from build123d import *

# Parameters (mm, degrees)
SALIENTE_EXTRUIR1_DEPTH = 6
REDONDEO1_R             = 10
REDONDEO2_R             = 5
REDONDEO3_R             = 1
CROQUIS2_R              = 1.803309478
CORTAR_EXTRUIR1_DEPTH   = 6
MATRIZL1_COUNT          = 2
MATRIZL1_PITCH          = 10
MATRIZL2_COUNT          = 2
MATRIZL2_PITCH          = 10


with BuildPart() as part:
    # Croquis1 → Saliente-Extruir1 (new body)
    with BuildSketch(Plane(origin=(0, 0, 0), x_dir=(1, 0, 0), z_dir=(0, 1, 0))):
        Polygon((0, -36.6), (0, -28.6), (7.646653433, -28.6), (7.646653433, -30.6), (22, -30.6), (22, -28.6), (22, 1.6), (22, 3.6), (9.500929434, 3.6), (9.500929434, 1.6), (0, 1.6), (0, 11.6), (30, 11.6), (30, -36.6), align=None)
    extrude(amount=SALIENTE_EXTRUIR1_DEPTH)

    # Redondeo1
    redondeo1_edges = [part.edges().sort_by_distance(p)[0] for p in [
        (30, 3, -11.6),
        (30, 3, 36.6),
    ]]
    fillet(redondeo1_edges, radius=REDONDEO1_R)

    # Redondeo2
    redondeo2_edges = [part.edges().sort_by_distance(p)[0] for p in [
        (22, 3, 30.6),
        (22, 3, -3.6),
    ]]
    fillet(redondeo2_edges, radius=REDONDEO2_R)

    # Redondeo3
    redondeo3_edges = [part.edges().sort_by_distance(p)[0] for p in [
        (0, 3, 28.6),
        (0, 3, -1.6),
    ]]
    fillet(redondeo3_edges, radius=REDONDEO3_R)

    # Croquis2 → Cortar-Extruir1 (cut)
    with BuildSketch(Plane(origin=(0, 6, 0), x_dir=(1, 0, 0), z_dir=(0, 1, 0))):
        with Locations(Location((26, -13.5, 0), (0, 0, 270))):
            Circle(CROQUIS2_R)
    cortar_extruir1 = extrude(amount=-CORTAR_EXTRUIR1_DEPTH, mode=Mode.SUBTRACT)

    # MatrizL1: Cortar-Extruir1 ×2
    with Locations(*[(0, 0, i * MATRIZL1_PITCH) for i in range(1, MATRIZL1_COUNT)]):
        add(cortar_extruir1, mode=Mode.SUBTRACT)

    # MatrizL2: Cortar-Extruir1 ×2
    with Locations(*[(0, 0, -i * MATRIZL2_PITCH) for i in range(1, MATRIZL2_COUNT)]):
        add(cortar_extruir1, mode=Mode.SUBTRACT)


solid = part.part
Build history of the part. All positions in model axes, mm. A direction names the side the tool comes from. Coordinates: 2 decimals unless noted, no trailing zeros. Order: outer loops, then holes, each group sorted by start corner. A loop starts at its lowest first (then second) coordinate and runs counter-clockwise, first axis right, second up. Notation, with made-up numbers: (2.5, 78.25) - (6.5, 78.25) arc R13 cw to (6.5, 83.25) - close; hole circle Ø3 at (49, 85). An arc over 180 degrees is marked (long way). Write item = value, one per line. Start each with the question number.
1) Wall check: line 1 along Z through (x, y) = (15.75, 4.3); line 2 along Z through (x, y) = (25, 5.2); line 3 along X through (y, z) = (2.05, 3.5). Give the ranges that are in metal, low to high. Write a range as from..to.
2) Saw through at B-B on y = 2.35. Write the cut outline in (x, z), then the cut area to 3 significant figures.
3) Saw through at C-C on x = 6. Write the cut outline in (y, z).
4) Saw through at A-A on x = 26. Write the cut outline in (y, z), then the cut area to 3 significant figures.
5) 3-axis set-ups, long thin cutter, end or side, ignore diameter. For faces 1 (the face through (0.301, 3.042, 28.885)), 2 (the face through (26.99, 3.04, -8.75)), 3 (the face through (13, 3, -3.6)): which of +Z, -Z, +X, -X, +Y, -Y reach the whole face in a straight line?
6) Saw through at D-D on z = 23.5. Write the cut outline in (x, y).
7) Flat gauge pins, fed straight in: pin 1 Ø3 at (x, y) = (25.5, 4) entering from +Z; pin 2 Ø6 at (x, z) = (12.5, 25) entering from -Y; pin 3 Ø3 at (y, z) = (2.5, 12.5) entering from -X; pin 4 Ø1.5 at (y, z) = (4, -1.5) entering from -X. Where does each tip first touch, or does it go through?
8) Two-plate mould, pull along X, no slides. Class faces 4 (the face through (22, 3, 13)), 5 (the face through (9.501, 3, -3)), 6 (the face through (25, 0, 7)): pulls with the +X half, pulls with the -X half, needs draft (parallel to the pull), parting line crosses it, or undercut.
From the geometry:
q1.line_1 = -11.6..-3.6, 30.6..36.6
q1.line_2 = -10.26..2, 5..12, 15..22, 25..35.26
q1.line_3 = 22..24.2, 27.8..30
q2.outline = (0, -11.6) - (20, -11.6) arc R10 ccw to (30, -1.6) - (30, 26.6) arc R10 ccw to (20, 36.6) - (0, 36.6) - (0, 29.6) arc R1 ccw to (1, 28.6) - (7.65, 28.6) - (7.65, 30.6) - (17, 30.6) arc R5 cw to (22, 25.6) - (22, 1.4) arc R5 cw to (17, -3.6) - (9.5, -3.6) - (9.5, -1.6) - (1, -1.6) arc R1 ccw to (0, -2.6) - close; hole circle Ø3.61 at (26, 3.5); hole circle Ø3.61 at (26, 13.5); hole circle Ø3.61 at (26, 23.5)
q2.area = 665 mm^2
q3.outline = (0, -11.6) - (6, -11.6) - (6, -1.6) - (0, -1.6) - close; (0, 28.6) - (6, 28.6) - (6, 36.6) - (0, 36.6) - close
q4.outline = (0, -9.6) - (6, -9.6) - (6, 1.7) - (0, 1.7) - close; (0, 5.3) - (6, 5.3) - (6, 11.7) - (0, 11.7) - close; (0, 15.3) - (6, 15.3) - (6, 21.7) - (0, 21.7) - close; (0, 25.3) - (6, 25.3) - (6, 34.6) - (0, 34.6) - close
q4.area = 200 mm^2
q5.face_1 = -X, +Y, -Y
q5.face_2 = -Z, +X, +Y, -Y
q5.face_3 = +Y, -Y
q6.outline = (22, 0) - (24.2, 0) - (24.2, 6) - (22, 6) - close; (27.8, 0) - (30, 0) - (30, 6) - (27.8, 6) - close
q7.pin_1 = 35.77
q7.pin_2 = through
q7.pin_3 = 22
q7.pin_4 = 0.06
q8.face_4 = pulls with the -X half
q8.face_5 = undercut
q8.face_6 = needs draft
